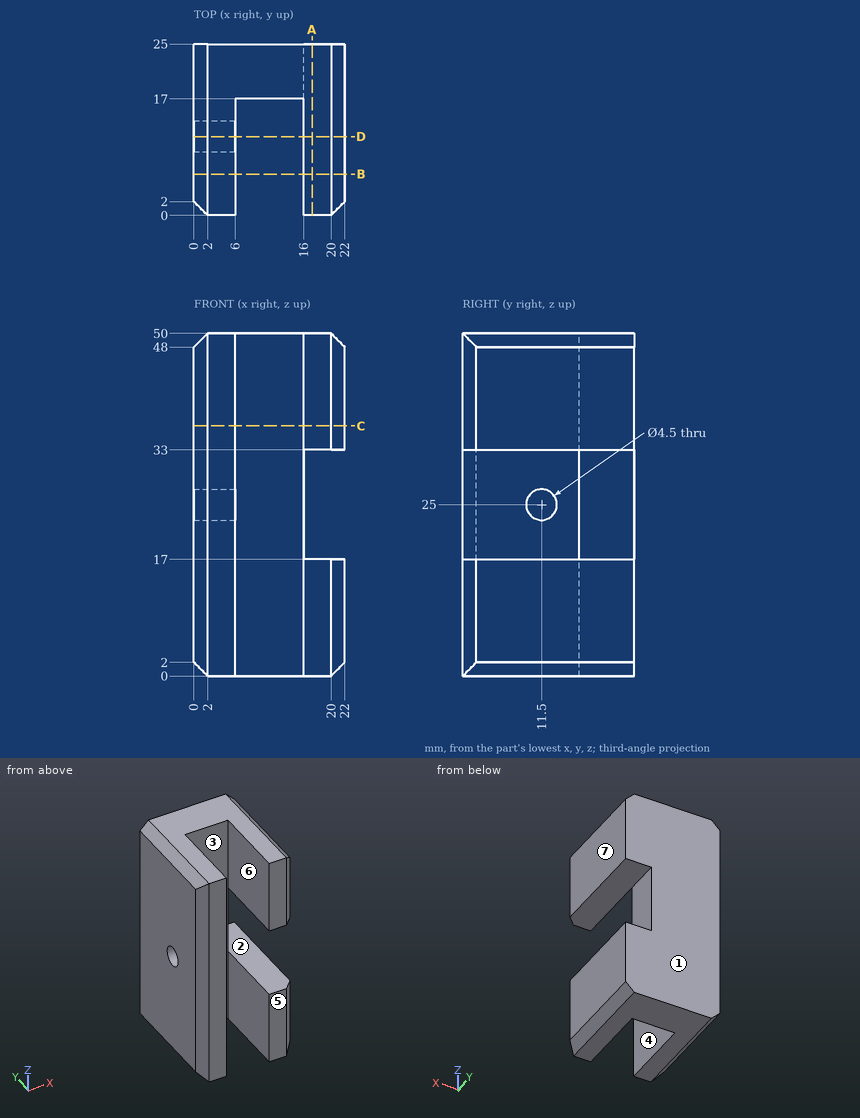
Input: dimensioned drawing with shaded views. Units: mm. Origin: part minimum x, y, z. A direction names the side the tool comes from. Give positions to 0.01 mm unless a question says otherwise; leave off trailing zeros. Write each loop counter-clockwise with the first axis right and the second up, starting at its lowest first coordinate (ties: lowest second). Pieces come first, ordered by that corner, then holes. Notation, with made-up numbers: (37.5, 9.25) -> (82.5, 9.25) arc R13 ccw to (82.5, 28.25) -> close; hole circle Ø10 at (77, -37). An arc over 180 degrees is marked (long way). Return JSON: item names as keys, results as strings. Group by question number.
1. Mould query, pull axis X, two halves, no side actions, for the marked faces 4, 5, 6 and 7. Classes: +X half, -X half, draft (parallel to the pull), parting line (faces both ways), or undercut.
2. Section C-C, the plane z = 36.5. Output: boundary loops of the cut face in (x, y).
3. Pin query (flat end, axial travel): pin 1 Ø6 at (x, z) = (11.5, 15) entering from -Y; pin 2 Ø9 at (y, z) = (23, 27.5) entering from +X. Return the tip coordinate at first contact, or that it passes through.
4. Section B-B, the plane y = 6. Output: boundary loops of the cut face in (x, z).
5. Section D-D, the plane y = 11.5. Output: boundary loops of the cut face in (x, z), then the cut area to 3 significant figures.
6. Access query for the marked faces 1, 2 and 3. Directions: +Z, -Z, +X, -X, +Y, -Y. A direction counts if a zero-diameter tool reaches every point of the face in a straight line with its end or side. Return the directions, or none.
7. Material intervals for line 1 (X direction, y = 8, z = 15); line 2 (Z direction, x = 3.9, y = 11.5); line 3 (Z direction, x = 17.25, y = 15), sorted ascending. Write a range as from..to.
8. Section A-A, the plane x = 17.25. Output: boundary loops of the cut face in (y, z), then the cut area to 3 significant figures.
Determined:
{
 "1": {"face 4": "undercut", "face 5": "draft", "face 6": "undercut", "face 7": "+X half"},
 "2": {"outline": "(0, 2) -> (2, 0) -> (6, 0) -> (6, 17) -> (16, 17) -> (16, 0) -> (20, 0) -> (22, 2) -> (22, 25) -> (0, 25) -> close"},
 "3": {"pin 1": "stops at y = 17", "pin 2": "stops at x = 16"},
 "4": {"outline": "(0, 2) -> (2, 0) -> (6, 0) -> (6, 50) -> (2, 50) -> (0, 48) -> close; (16, 0) -> (20, 0) -> (22, 2) -> (22, 17) -> (16, 17) -> close; (16, 33) -> (22, 33) -> (22, 48) -> (20, 50) -> (16, 50) -> close"},
 "5": {"outline": "(0, 2) -> (2, 0) -> (6, 0) -> (6, 22.75) -> (0, 22.75) -> close; (0, 27.25) -> (6, 27.25) -> (6, 50) -> (2, 50) -> (0, 48) -> close; (16, 0) -> (20, 0) -> (22, 2) -> (22, 17) -> (16, 17) -> close; (16, 33) -> (22, 33) -> (22, 48) -> (20, 50) -> (16, 50) -> close", "area": "469 mm2"},
 "6": {"face 1": "+Z, -Z, +X, -X, +Y", "face 2": "+X, +Y, -Y", "face 3": "+Z, -Z, -Y"},
 "7": {"line 1": "x = 0..6, 16..22", "line 2": "z = 0..22.75, 27.25..50", "line 3": "z = 0..17, 33..50"},
 "8": {"outline": "(0, 0) -> (25, 0) -> (25, 17) -> (0, 17) -> close; (0, 33) -> (25, 33) -> (25, 50) -> (0, 50) -> close", "area": "850 mm2"}
}
